CAD build for the part. Positions are in the model's coordinates, mm. A direction names the side the tool comes from. Coordinates: 2 decimals unless noted, no trailing zeros. Write each loop counter-clockwise with the first axis right and the second up, starting at its lowest first coordinate (ties: lowest second). Pieces come first, ordered by that corner, then holes. Notation, with made-up numbers: (66.25, -19.5) -> (97.25, -19.5) arc R28 ccw to (97.25, 4.5) -> close; hole circle Ø10 at (12, 76). An arc over 180 degrees is marked (long way). Answer as CSV lines item,"result". Start each with the question number.
```python
from build123d import *

# Parameters (mm, degrees)
F0_R      = 7
F1_DEPTH  = 2
F2_R      = 9
F2_R_2    = 7
F3_DEPTH  = 2
F3_FACE_R = 9
F5_R      = 2.5
F10_DEPTH = 5


with BuildPart() as f1:
    # F0 (on Top) → F1 (new body)
    with BuildSketch(Plane.XY):
        Circle(F0_R)
    extrude(amount=F1_DEPTH)

    # F2 (on face) → F3 (join)
    with BuildSketch(Plane.XY.offset(2)):
        Circle(F2_R)
        Circle(F2_R_2, mode=Mode.SUBTRACT)
        Circle(F2_R_2)
    extrude(amount=F3_DEPTH)

    # F3_face (on face) → F6 section 0
    with BuildSketch(Plane.XY.offset(4)):
        Circle(F3_FACE_R)
    # F5 (on offset) → F6 section 1
    with BuildSketch(Plane.XY.offset(29)):
        Circle(F5_R)
    loft()

    # F7 (on face) → F8 (revolve)
    with BuildSketch(Plane.XY.offset(29)):
        with BuildLine():
            Line((2.5, 0), (5, 0))
            ThreePointArc((5, 0), (0, 5), (-5, 0))
            Line((-5, 0), (-2.5, 0))
            ThreePointArc((-2.5, 0), (0, 2.5), (2.5, 0))
        make_face()
        with BuildLine():
            ThreePointArc((-2.5, 0), (0, -2.5), (2.5, 0))
            Line((2.5, 0), (-2.5, 0))
        make_face()
    revolve(axis=Axis((0, 0, 29), (1, 0, 0)))

    # F9 (on face) → F10 (join)
    with BuildSketch(Plane(origin=(0, 0, 2), x_dir=(1, 0, 0), z_dir=(0, 0, -1))):
        with BuildLine():
            ThreePointArc((1.4947825929, 8.875), (0, 9), (-1.4947825929, 8.875))
            ThreePointArc((-1.4947825929, 8.875), (0, 7.5), (1.4947825929, 8.875))
        make_face()
        with BuildLine():
            ThreePointArc((1.4947825929, 8.875), (1.4986950806, 8.937445581), (1.5, 9))
            ThreePointArc((1.5, 9), (-0.062554419, 10.4986950806), (-1.4947825929, 8.875))
            ThreePointArc((-1.4947825929, 8.875), (0, 9), (1.4947825929, 8.875))
        make_face()
        with BuildLine():
            ThreePointArc((-6.2942286341, -4.5), (-6.9907073778, -3.2333691972), (-8.433366755, -3.1429803014))
            ThreePointArc((-8.433366755, -3.1429803014), (-7.7942286341, -4.5), (-6.9385841621, -5.7320196986))
            ThreePointArc((-6.9385841621, -5.7320196986), (-6.4650434122, -5.1951738244), (-6.2942286341, -4.5))
        make_face()
        with BuildLine():
            ThreePointArc((-6.9385841621, -5.7320196986), (-7.7942286341, -4.5), (-8.433366755, -3.1429803014))
            ThreePointArc((-8.433366755, -3.1429803014), (-9.0932667397, -5.25), (-6.9385841621, -5.7320196986))
        make_face()
        with BuildLine():
            ThreePointArc((6.9385841621, -5.7320196986), (7.7942286341, -4.5), (8.433366755, -3.1429803014))
            ThreePointArc((8.433366755, -3.1429803014), (6.4951905284, -3.75), (6.9385841621, -5.7320196986))
        make_face()
        with BuildLine():
            ThreePointArc((9.2942286341, -4.5), (9.0608594369, -3.6964787437), (8.433366755, -3.1429803014))
            ThreePointArc((8.433366755, -3.1429803014), (7.7942286341, -4.5), (6.9385841621, -5.7320196986))
            ThreePointArc((6.9385841621, -5.7320196986), (8.4894024584, -5.8291852218), (9.2942286341, -4.5))
        make_face()
    extrude(amount=-F10_DEPTH)


solid = f1.part
```
1. Flat gauge pins, fed straight in: P1, Ø2.5, axis at x = 8.5, y = 5, coming from the +Z side; P2, Ø8, axis at x = -2, y = -6.5, coming from the -Z side; P3, Ø3, axis at x = 1.5, y = -8.5, coming from the -Z side; P4, Ø8, axis at y = -3.5, z = 24, coming from the -X side. Where does each tip first touch, or does it go through?
2. Mould opens along Z. For faces 1 (the face through (-8, 4, 7)), 2 (the face through (-1.206, -5.433, 17.212)), 3 (the face through (7.738, -4.596, 2.986)), 4 (the face through (0, 0, 0)) say: pulls with the +Z half, pulls with the -Z half, needs draft (parallel to the pull), parting line crosses it, or undercut.
3. Cut at A-A (z = 14). Give the cut face in (x, y), then the cut area to 3 significant figures.
4. Tool access for faces 5 (the face through (3, 7, 2)), 6 (the face through (0, 9, 3)), 7 (the face through (8, 4, 7)): list every direction of +Z, -Z, +X, -X, +Y, -Y with a clear straight run to the whole face (end or side of a thin tool).
5. Wall check: line 1 (Y direction, x = 2.5, z = 15.5); line 2 (X direction, y = -3.25, z = 26); line 3 (X direction, y = -5.5, z = 9.5). Give the ranges that are in metal, low to high.
6. Cut at C-C (z = 31). Give the cut face in (x, y).
7. Cut at B-B (x = 0). Give the cut face in (y, z), then the cut area to 3 significant figures.
Geometry check:
1,P1,"z = 7"
1,P2,"z = 0"
1,P3,"z = 2"
1,P4,"x = -4.54"
2,face 1,"pulls with the +Z half"
2,face 2,"undercut"
2,face 3,"needs draft"
2,face 4,"pulls with the -Z half"
3,outline,"circle Ø12.8 at (0, 0)"
3,area,"129 mm²"
4,face 5,"-Z"
4,face 6,"+Z, -Z, +Y"
4,face 7,"+Z, +X, +Y"
5,line 1,"-5.47 to 5.47"
5,line 2,"-2.33 to 2.33"
5,line 3,"-5.2 to 5.2"
6,outline,"circle Ø9.17 at (0, 0)"
7,outline,"(-10.5, 2) -> (-7, 2) -> (-7, 0) -> (7, 0) -> (7, 2) -> (9, 2) -> (9, 4) -> (3.44, 25.37) arc R5 ccw (long way) to (-3.44, 25.37) -> (-8.22, 7) -> (-10.5, 7) -> close"
7,area,"411 mm²"
